Here's how the part is built. I have some questions about the finished solid (model axes, mm). Face numbers are marked on the shaded views. A direction names the side the tool comes from. Give positions to 0.01 mm unless a question says otherwise; leave off trailing zeros. Loops run counter-clockwise (first coordinate to the right, second up) from the corner with the lowest first, then second, coordinate; pieces in that order, holes last.
Q1. For the marked faces 1 and 2, which set-ups out of +Z, -Z, +X, -X, +Y, -Y let a thin tool reach every point of the face, with its end or its side?
Q2. If we section it at C-C (z = 12.7): Please give me the cut outline in (x, y).
Q3. If we section it at A-A (x = -139.7): Please give me the cut outline in (y, z).
Q4. I need wall thicknesses on line 1 (Y direction, x = -13, z = 12.7); line 2 (Z direction, x = -140, y = -33.5); line 3 (Y direction, x = -48, z = 17.5). Which ranges of each line are inside material? Lowest first, please.
Q5. If we section it at B-B (y = -35.5): Please give me the cut outline in (x, z), plus the area to 3 significant figures.
Q6. If we section it at D-D (x = -42): Please give me the cut outline in (y, z), plus the area to 3 significant figures.
Q7. Will these pins go through, and if not, where does the flat tip stop? P1, Ø14.5, axis at y = 105.83, z = 12.7, coming from the -X side; P2, Ø8, axis at x = -116, z = 7.5, coming from the +Y side; P3, Ø10, axis at y = 48.5, z = 13, coming from the -X side.
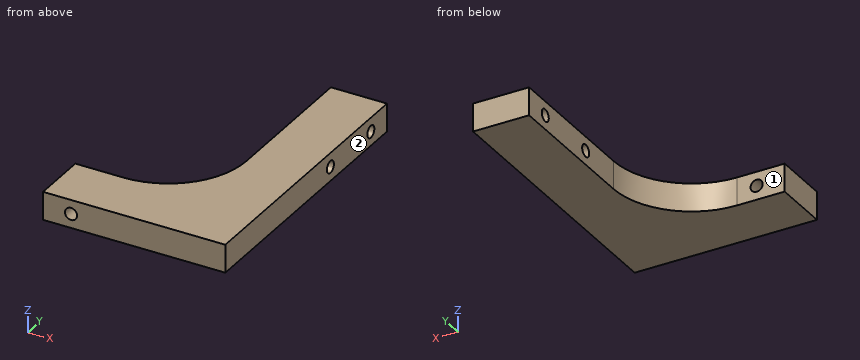
from build123d import *

# Parameters (mm, degrees)
BOSS_EXTRUDE1_DEPTH   = 25.4
M10_CLEARANCE_HOLE1_D = 11
M10_CLEARANCE_HOLE2_D = 11
FILLET1_R             = 70.96


with BuildPart() as part:
    # Sketch1 → Boss-Extrude1 (new body)
    with BuildSketch(Plane.XY):
        Polygon((0, 194.731808123), (0, -59.268191877), (-165.1, -59.268191877), (-165.1, -8.468191877), (-50.8, -8.468191877), (-50.8, 194.731808123), align=None)
    extrude(amount=BOSS_EXTRUDE1_DEPTH)

    # M10 Clearance Hole1 (through all)
    with Locations(Plane(origin=(0, -8.468191877, 0), x_dir=(1, 0, 0), z_dir=(0, 1, 0))):
        with Locations((-139.7, -12.7)):
            Hole(M10_CLEARANCE_HOLE1_D / 2)

    # M10 Clearance Hole2 (through all)
    with Locations(Plane.ZY.offset(50.8)):
        with Locations((12.7, 169.331808123), (12.7, 105.831808123)):
            Hole(M10_CLEARANCE_HOLE2_D / 2)

    # Fillet1
    fillet1_edges = [part.edges().sort_by_distance(p)[0] for p in [
        (-50.8, -8.468191877, 12.7),
    ]]
    fillet(fillet1_edges, radius=FILLET1_R)


solid = part.part
Check sheet entries:
1. face 1: +Z, -Z, -X, +Y
1. face 2: +Z, -Z, +X, +Y, -Y
2. outline: (-165.1, -59.27) - (-145.2, -59.27) - (-145.2, -8.47) - (-165.1, -8.47) - close; (-134.2, -59.27) - (0, -59.27) - (0, 100.33) - (-50.8, 100.33) - (-50.8, 62.49) arc R70.96 cw to (-121.76, -8.47) - (-134.2, -8.47) - close; (-50.8, 111.33) - (0, 111.33) - (0, 163.83) - (-50.8, 163.83) - close; (-50.8, 174.83) - (0, 174.83) - (0, 194.73) - (-50.8, 194.73) - close
3. outline: (-59.27, 0) - (-8.47, 0) - (-8.47, 7.2) - (-59.27, 7.2) - close; (-59.27, 18.2) - (-8.47, 18.2) - (-8.47, 25.4) - (-59.27, 25.4) - close
4. line 1: y = -59.27 to 100.33, 111.33 to 163.83, 174.83 to 194.73
4. line 2: z = 0 to 7.21, 18.19 to 25.4
4. line 3: y = -59.27 to 103.15, 108.52 to 166.65, 172.02 to 194.73
5. outline: (-165.1, 0) - (0, 0) - (0, 25.4) - (-165.1, 25.4) - close; hole circle Ø11 at (-139.7, 12.7)
5. area: 4,100 mm2
6. outline: (-59.27, 0) - (194.73, 0) - (194.73, 25.4) - (-59.27, 25.4) - close; hole circle Ø11 at (105.83, 12.7); hole circle Ø11 at (169.33, 12.7)
6. area: 6,260 mm2
7. P1: stops at x = -50.8
7. P2: stops at y = -7.79
7. P3: stops at x = -53.39
